Design review of the part built by this model. Coordinates are the model's own, in mm. A direction names the side the tool comes from. Round coordinates to 2 decimals unless told otherwise and drop trailing zeros. Order: outer loops, then holes, each group sorted by start corner. A loop starts at its lowest first (then second) coordinate and runs counter-clockwise, first axis right, second up. Notation, with made-up numbers: (66, -32) - (120, -32) arc R16 ccw to (120, -16) - close; hole circle Ø5 at (-35.75, 65). An arc over 180 degrees is marked (long way). Answer as a JSON object with one key per item and string values. Group by question number.
from build123d import *

# Parameters (mm, degrees)
SKETCH1_R           = 16
BOSS_EXTRUDE1_DEPTH = 10
CHAMFER1_SIZE       = 3
FILLET1_R           = 3
SKETCH2_R           = 2.65
CUT_EXTRUDE1_DEPTH  = 10
SKETCH3_R           = 15
CUT_EXTRUDE2_DEPTH  = 5


with BuildPart() as part:
    # Sketch1 → Boss-Extrude1 (new body)
    with BuildSketch(Plane(origin=(0, 0, 0), x_dir=(1, 0, 0), z_dir=(0, 1, 0))):
        with Locations(Location((0, 0, 0), (0, 0, 270))):
            Circle(SKETCH1_R)
    extrude(amount=BOSS_EXTRUDE1_DEPTH)

    # Chamfer1
    chamfer1_edges = [part.edges().sort_by_distance(p)[0] for p in [
        (0, 10, -16),
    ]]
    chamfer(chamfer1_edges, length=CHAMFER1_SIZE)

    # Fillet1
    fillet1_edges = [part.edges().sort_by_distance(p)[0] for p in [
        (0, 10, -13),
        (0, 7, -16),
    ]]
    fillet(fillet1_edges, radius=FILLET1_R)

    # Sketch2 → Cut-Extrude1 (cut)
    with BuildSketch(Plane(origin=(0, 10, 0), x_dir=(1, 0, 0), z_dir=(0, 1, 0))):
        with Locations(Location((0, 0, 0), (0, 0, 270))):
            Circle(SKETCH2_R)
    extrude(amount=-CUT_EXTRUDE1_DEPTH, mode=Mode.SUBTRACT)

    # Sketch3 → Cut-Extrude2 (cut)
    with BuildSketch(Plane.XZ):
        with Locations(Location((0, 0, 0), (0, 0, 270))):
            Circle(SKETCH3_R)
    extrude(amount=-CUT_EXTRUDE2_DEPTH, mode=Mode.SUBTRACT)


solid = part.part
1. To check wall thickness, follow line 1 (X direction, y = 3.35, z = 0); line 2 (Z direction, x = 7, y = 1.75); line 3 (Y direction, x = 3.5, z = 7.5). State the ranges of each line that lie inside material, in increasing order. Write a range as from..to.
2. Take a section at B-B, the plane y = 1.25. Give the boundary of the cut face in (x, z), then the cut area to 3 significant figures.
3. Clearance check with flat-ended pins moving along their axes: P1, Ø2, axis at x = 1.5, y = 6.5, coming from the +Z side; P2, Ø2, axis at x = -10.5, y = 6.5, coming from the -Z side; P3, Ø5, axis at x = 11.5, z = -2.5, coming from the -Y side. State where each tip first meets the part, or that it passes through.
4. Take a section at A-A, the plane y = 8.75. Give the boundary of the cut face in (x, z).
5. Tool access review of faces 1 (the cylindrical face through (0.66, 2.465, 14.985)), 2 (the cylindrical face through (-1.612, 7.535, -2.103)): name each direction out of +Z, -Z, +X, -X, +Y, -Y from which nothing blocks a thin tool from reaching the whole face with its end or side.
Response values:
{
 "1": {"line 1": "-16..-15, 15..16", "line 2": "-14.39..-13.27, 13.27..14.39", "line 3": "5..10"},
 "2": {"outline": "circle Ø32 at (0, 0); hole circle Ø30 at (0, 0)", "area": "97.4 mm2"},
 "3": {"P1": "z = 15.98", "P2": "z = -12.8", "P3": "y = 5"},
 "4": {"outline": "circle Ø28.5 at (0, 0); hole circle Ø5.3 at (0, 0)"},
 "5": {"face 1": "-Y", "face 2": "+Y, -Y"}
}
